CAD build for the part. Positions are in the model's coordinates, mm. A direction names the side the tool comes from. Coordinates: 2 decimals unless noted, no trailing zeros. Loops run counter-clockwise (first coordinate to the right, second up) from the corner with the lowest first, then second, coordinate; pieces in that order, holes last. Notation, with made-up numbers: (18, -11.5) -> (32, -11.5) arc R25 cw to (32, 8.5) -> close; hole circle Ø3 at (37, 61). An arc over 180 degrees is marked (long way). Answer as a JSON object with one key per item and string values. Group by question number.
from build123d import *

# Parameters (mm, degrees)
SKETCH_1_W          = 20
SKETCH_1_H          = 20
EXTRUDE_2_DEPTH     = 8
SKETCH_2_W          = 5
SKETCH_2_H          = 12
EXTRUDE_3_DEPTH     = 51
CUT_EXTRUDE_1_DEPTH = 63.104750221


with BuildPart() as part:
    # 草图1 → 凸台-拉伸2 (new body)
    with BuildSketch(Plane.XY):
        Rectangle(SKETCH_1_W, SKETCH_1_H)
        with BuildLine():
            Line((6.708203932, -2), (9, -2))
            Line((9, -2), (9, 2))
            Line((9, 2), (6.708203932, 2))
            ThreePointArc((6.708203932, 2), (-7, 0), (6.708203932, -2))
        make_face(mode=Mode.SUBTRACT)
    extrude(amount=EXTRUDE_2_DEPTH)

    # 草图2 → 凸台-拉伸3 (add)
    with BuildSketch(Plane(origin=(10, 0, 0), x_dir=(0, 0, -1), z_dir=(1, 0, 0))):
        with Locations((-4.5, 0)):
            Rectangle(SKETCH_2_W, SKETCH_2_H)
    extrude(amount=EXTRUDE_3_DEPTH)

    # 草图3 → 切除-拉伸1 (cut, through all)
    with BuildSketch(Plane(origin=(0, 0, 2), x_dir=(-1, 0, 0), z_dir=(0, 0, -1))):
        with BuildLine():
            Line((-56.5, 3), (-36.5, 3))
            ThreePointArc((-36.5, 3), (-33.5, 0), (-36.5, -3))
            Line((-36.5, -3), (-56.5, -3))
            ThreePointArc((-56.5, -3), (-59.5, 0), (-56.5, 3))
        make_face()
    extrude(amount=-CUT_EXTRUDE_1_DEPTH, mode=Mode.SUBTRACT)


solid = part.part
Item 1: Drill centre lines: L1, parallel to X at y = 0, z = 2.25; L2, parallel to Y at x = 0, z = 2.25; L3, parallel to Y at x = 45.5, z = 5. Where is each one in solid material? Low to high.
Item 2: Band-saw the part on C-C, the plane z = 5.25. List the corners of the cut face in (x, y), and give its area (3 significant figures).
Item 3: Pull direction Y, two halves, no side cores. Call faces 1 (the flat face through (0, 10, 4)), 2 (the flat face through (47, 3, 4)), 3 (the flat face through (61, 0, 5)): +Y half, -Y half, draft (parallel to the pull), parting line (faces both ways), or undercut.
Item 4: Flat gauge pins, fed straight in: P1, Ø8, axis at x = 34, y = 7, coming from the -Z side; P2, Ø11, axis at x = 0, y = 0, coming from the +Z side; P3, Ø3, axis at x = 31, y = -5, coming from the +Z side; P4, Ø1.5, axis at x = 30.5, z = 4.5, coming from the -Y side. Where does each tip first touch, or does it go through?
Item 5: 3-axis set-ups, long thin cutter, end or side, ignore diameter. For faces 4 (the flat face through (35, 6, 5)), 5 (the flat face through (35, -6, 5)), 6 (the flat face through (46, -3, 4)): which of +Z, -Z, +X, -X, +Y, -Y reach the whole face in a straight line?
Item 6: Band-saw the part on D-D, the plane x = 51. List the corners of the cut face in (y, z).
Item 7: Band-saw the part on A-A, the plane y = 0. List the corners of the cut face in (x, z), and give its area (3 significant figures).
Item 8: Band-saw the part on B-B, the plane x = 0. List the corners of the cut face in (y, z).
Reply:
{
 "1": {"L1": "-10 to -7, 9 to 33.5, 59.5 to 61", "L2": "-10 to -7, 7 to 10", "L3": "-6 to -3, 3 to 6"},
 "2": {"outline": "(-10, -10) -> (10, -10) -> (10, -6) -> (61, -6) -> (61, 6) -> (10, 6) -> (10, 10) -> (-10, 10) -> close; hole (6.71, -2) -> (9, -2) -> (9, 2) -> (6.71, 2) arc R7 ccw (long way) to start; hole (36.5, -3) -> (56.5, -3) arc R3 ccw to (56.5, 3) -> (36.5, 3) arc R3 ccw to start", "area": "701 mm²"},
 "3": {"face 1": "+Y half", "face 2": "undercut", "face 3": "draft"},
 "4": {"P1": "z = 2", "P2": "through", "P3": "z = 7", "P4": "y = -6"},
 "5": {"face 4": "+Z, -Z, +X, +Y", "face 5": "+Z, -Z, +X, -Y", "face 6": "+Z, -Z"},
 "6": {"outline": "(-6, 2) -> (-3, 2) -> (-3, 7) -> (-6, 7) -> close; (3, 2) -> (6, 2) -> (6, 7) -> (3, 7) -> close"},
 "7": {"outline": "(-10, 0) -> (-7, 0) -> (-7, 8) -> (-10, 8) -> close; (9, 0) -> (10, 0) -> (10, 2) -> (33.5, 2) -> (33.5, 7) -> (10, 7) -> (10, 8) -> (9, 8) -> close; (59.5, 2) -> (61, 2) -> (61, 7) -> (59.5, 7) -> close", "area": "157 mm²"},
 "8": {"outline": "(-10, 0) -> (-7, 0) -> (-7, 8) -> (-10, 8) -> close; (7, 0) -> (10, 0) -> (10, 8) -> (7, 8) -> close"}
}
